Check sheet for the drawn part. Datum: minimum x, y, z corner. Units: mm. Coordinates: 2 decimals unless noted, no trailing zeros. Order: outer loops, then holes, each group sorted by start corner. A loop starts at its lowest first (then second) coordinate and runs counter-clockwise, first axis right, second up.
1. Gauge pin test, flat ends, axial feed: pin 1 Ø2.5 at (x, y) = (57, 1.5) entering from -Z; pin 2 Ø12 at (x, y) = (57, 16.5) entering from -Z; pin 3 Ø0.9 at (x, y) = (3, 28.5) entering from -Z. Record the tip position at first contact, or that the pin passes through.
2. Cross-section at B-B (z = 53). Enter the section's corners in (x, y).
3. Draft check along Y on the marked faces 1, 2, 3 and 4. Enter one of: released by +Y, released by -Y, zero draft, split by the parting line, or undercut.
4. Thickness scan on line 1 (Y direction, x = 16, z = 69); line 2 (X direction, y = 21, z = 90.5); line 3 (Z direction, x = 51, y = 15). Record the ranges inside material, lowest first.
5. Cross-section at D-D (x = 83). Enter the section's corners in (y, z), then the cut area to 3 significant figures.
6. Cross-section at C-C (y = 25). Enter the section's corners in (x, z), then the cut area to 3 significant figures.
7. Cross-section at A-A (x = 10.5). Enter the section's corners in (y, z).
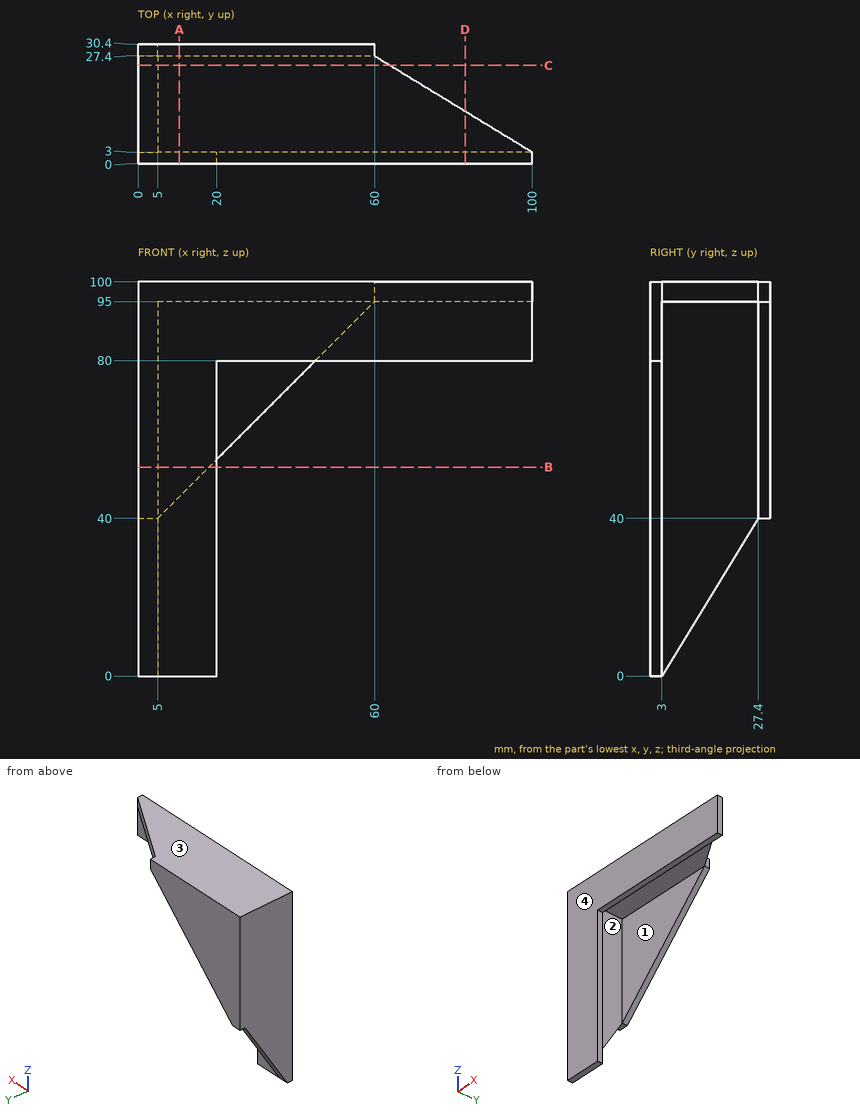
Data:
1. pin 1: stops at z = 80
1. pin 2: stops at z = 95
1. pin 3: stops at z = 40
2. outline: (0, 0) - (20, 0) - (20, 3) - (5, 3) - (5, 27.4) - (18, 27.4) - (18, 30.4) - (0, 30.4) - close
3. face 1: undercut
3. face 2: undercut
3. face 3: zero draft
3. face 4: released by -Y
4. line 1: y = 0 to 3, 27.4 to 30.4
4. line 2: x = 0 to 5
4. line 3: z = 95 to 100
5. outline: (0, 80) - (3, 80) - (3, 95) - (13.37, 95) - (13.37, 100) - (0, 100) - close
5. area: 112 mm2
6. outline: (0, 36.07) - (5, 36.07) - (5, 95) - (63.93, 95) - (63.93, 100) - (0, 100) - close
6. area: 614 mm2
7. outline: (0, 0) - (3, 0) - (3, 95) - (27.4, 95) - (27.4, 45.5) - (30.4, 45.5) - (30.4, 100) - (0, 100) - close
